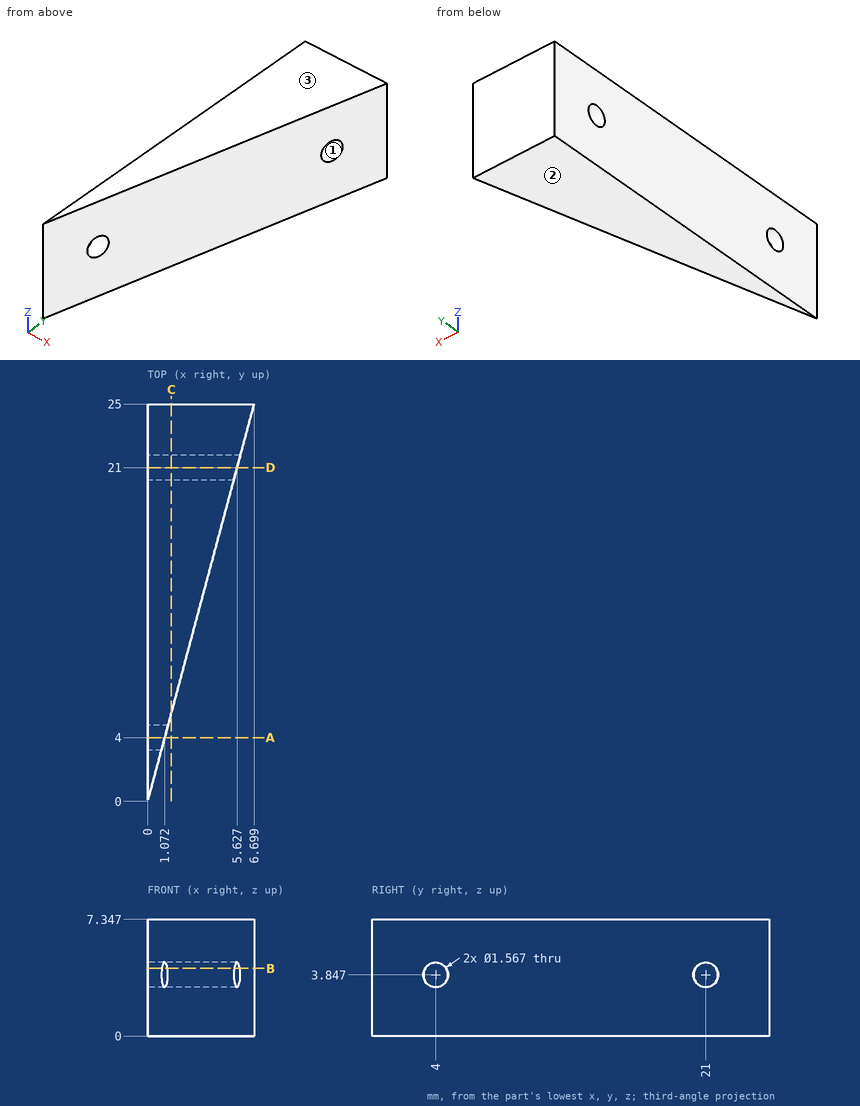
Verification items for this drawing (mm, ordinates from the low corner). Coordinates: 2 decimals unless noted, no trailing zeros. Write each loop counter-clockwise with the first axis right and the second up, starting at its lowest first coordinate (ties: lowest second). Pieces come first, ordered by that corner, then holes. Notation, with made-up numbers: M 71.5,47 L 84.5,47 A34 ccw 84.5,81 Z; hole C 47.25,0 d11. An arc over 180 degrees is marked long. Use one line per item in the form item = value. Start each with the question number.
1) Go/stop test with flat-tipped pins: pin 1 Ø3 at (x, y) = (2, 21.5) entering from -Z; pin 2 Ø2 at (y, z) = (21, 3.847) entering from +X (1 decimal). Record where each tip stops, or that it passes through.
2) Release check for a two-part mould opening along Z. For the marked faces 1, 2 and 3 record: pulls with the +Z half, pulls with the -Z half, needs draft (parallel to the pull), parting line crosses it, or undercut.
3) Section check C-C on x = 1.5. Enter the section's corners in (y, z).
4) Section check D-D on y = 21. Enter the section's corners in (x, z), and give its area (3 significant figures).
5) Thickness scan on probe 1 along Z at (x, y) = (0.85, 4); probe 2 along X at (y, z) = (11, 3.5); probe 3 along X at (y, z) = (7.25, 1.5). Record the ranges inside material, lowest first. Write a range as from..to.
6) Section check A-A on y = 4. Enter the section's corners in (x, z).
7) Section check B-B on z = 4.25. Enter the section's corners in (x, y).
Responses:
q1.pin_1 = 0
q1.pin_2 = 5.9
q2.face_1 = undercut
q2.face_2 = pulls with the -Z half
q2.face_3 = pulls with the +Z half
q3.outline = M 5.6,0 L 25,0 L 25,7.35 L 5.6,7.35 Z; hole C 21,3.85 d1.57
q4.outline = M 0,0 L 5.63,0 L 5.63,3.06 L 0,3.06 Z; M 0,4.63 L 5.63,4.63 L 5.63,7.35 L 0,7.35 Z
q4.area = 32.5 mm2
q5.probe_1 = 0..3.06, 4.63..7.35
q5.probe_2 = 0..2.95
q5.probe_3 = 0..1.94
q6.outline = M 0,0 L 1.07,0 L 1.07,3.06 L 0,3.06 Z; M 0,4.63 L 1.07,4.63 L 1.07,7.35 L 0,7.35 Z
q7.outline = M 0,0 L 0.89,3.33 L 0,3.33 Z; M 0,4.67 L 1.25,4.67 L 5.45,20.33 L 0,20.33 Z; M 0,21.67 L 5.81,21.67 L 6.7,25 L 0,25 Z
